Geometry check sheet. Reference: the model listing, model coordinates, mm. Round coordinates to 2 decimals unless told otherwise and drop trailing zeros. Order: outer loops, then holes, each group sorted by start corner. A loop starts at its lowest first (then second) coordinate and runs counter-clockwise, first axis right, second up. Notation, with made-up numbers: (68.5, 27) - (91.5, 27) arc R10 cw to (91.5, 37) - close; hole circle Ø2 at (-9, 11.25). An arc over 180 degrees is marked (long way). Return JSON: item names as keys, results as strings. Group by question number.
Q1. Sectioned sample at A-A, the plane z = -10.5. Record the cut outline in (x, y).
Q2. Sectioned sample at B-B, the plane x = -22.5. Record the cut outline in (y, z), then the cut area to 3 significant figures.
Q3. Gauge pin test, flat end, axial feed: pin 1 Ø2 at (x, z) = (13.644, -6.75) entering from +Y. Record the tip position at first contact, or that the pin passes through.
Q4. Sectioned sample at C-C, the plane y = 0.7. Record the cut outline in (x, z).
Q5. Sectioned sample at D-D, the plane x = -31.5. Record the cut outline in (y, z).
Q6. Material ranges on line 1 along X through (y, z) = (1.65, -6.75); line 2 along Z through (x, y) = (-22.4, 0.6); line 3 along X through (y, z) = (0.9, -3), recorded low to high.
Autodesk Inventor part; units mm, degrees
ref_plane "YZ Plane" through (0, 0, 0) normal (1, 0, 0) x (0, 1, 0)
ref_plane "XZ Plane" through (0, 0, 0) normal (0, 1, 0) x (-1, 0, 0)
ref_plane "XY Plane" through (0, 0, 0) normal (0, 0, 1) x (1, 0, 0)
sketch "Sketch1" plane through (0, 0, 0) normal (0, 1, 0) x (-1, 0, 0)
  line L0 (0, 0) -> (32.4, 0)
  line L1 (32.4, 0) -> (32.4, -13.5)
  line L2 (32.4, -13.5) -> (0, -13.5)
  line L3 (0, -13.5) -> (0, 0)
  line L4 (-5, 5) -> (37.4, 5)
  line L5 (37.4, 5) -> (37.4, -18.5)
  line L6 (37.4, -18.5) -> (-5, -18.5)
  line L7 (-5, -18.5) -> (-5, 5)
  line L8 (37.4, 5) -> (-5, 21.2758)
  line L9 (-5, 21.2758) -> (-5, -34.7758)
  line L10 (-5, -34.7758) -> (37.4, -18.5)
  line L11 (-5, 21.2758) -> (-8.0516, 15.5367)
  line L12 (-8.0516, 15.5367) -> (-17.644, 5.25)
  line L13 (-17.644, 5.25) -> (-17.644, -18.75)
  line L14 (-17.644, -18.75) -> (-8.0516, -29.0367)
  line L15 (-8.0516, -29.0367) -> (-5, -34.7758)
  point P0 (-5, -6.75)
  dimension "d0" = 32.4
  dimension "d1" = 13.5
  dimension "d2" = 5
  dimension "d5" = 21
  dimension "d6" = 21
  dimension "d8" = 28
  dimension "d9" = 28
  dimension "d11" = 6.5
  dimension "d12" = 24
  dimension "d13" = 6.5
  dimension "d15" = 165
  dimension "d16" = 165
extrude "Extrusion1" add sketch "Sketch1" along normal blind 2
fillet "Fillet1" radius 3 8 edges at (5, 1, 21.2758) (17.644, 1, 5.25) (17.644, 1, -18.75) (5, 1, -34.7758) (8.0516, 1, -29.0367) (8.0516, 1, 15.5367) (-37.4, 1, 5) (-37.4, 1, -18.5)
sketch "Sketch2" plane through (0, 2, 0) normal (0, 1, 0) x (1, 0, 0)
  circle A0 centre (3.1296, -16.2733) radius 1.1
  circle A1 centre (3.1296, 29.7733) radius 1.1
  circle A2 centre (13.644, 6.75) radius 1.1
  circle A3 centre (-22.4, -6.4734) radius 1.1
  circle A4 centre (-22.4, 19.9734) radius 1.1
  arc A5 (-35.4751, 19.2389) -> (-37.4, 16.4382) centre (-34.4, 16.4382) ccw
  line L0 (-37.4, 16.4382) -> (-37.4, -2.9382)
  arc A6 (-37.4, -2.9382) -> (-35.4751, -5.7389) centre (-34.4, -2.9382) ccw
  line L1 (-35.4751, -5.7389) -> (2.5221, -20.3247)
  arc A7 (2.5221, -20.3247) -> (6.2461, -18.9323) centre (3.5972, -17.5239) ccw
  line L2 (6.2461, -18.9323) -> (7.8661, -15.8854)
  arc A8 (8.3209, -15.2478) -> (7.8661, -15.8854) centre (10.515, -17.2938) ccw
  line L3 (8.3209, -15.2478) -> (16.8381, -6.1143)
  arc A9 (16.8381, -6.1143) -> (17.644, -4.0683) centre (14.644, -4.0683) ccw
  line L4 (17.644, -4.0683) -> (17.644, 17.5683)
  arc A10 (17.644, 17.5683) -> (16.8381, 19.6143) centre (14.644, 17.5683) ccw
  line L5 (16.8381, 19.6143) -> (8.3209, 28.7478)
  arc A11 (7.8661, 29.3854) -> (8.3209, 28.7478) centre (10.515, 30.7938) ccw
  line L6 (7.8661, 29.3854) -> (6.2461, 32.4323)
  arc A12 (6.2461, 32.4323) -> (2.5221, 33.8247) centre (3.5972, 31.0239) ccw
  line L7 (2.5221, 33.8247) -> (-35.4751, 19.2389)
  line L8 (0, 0) -> (-32.4, 0)
  line L9 (-32.4, 0) -> (-32.4, 13.5)
  line L10 (-32.4, 13.5) -> (0, 13.5)
  line L11 (0, 13.5) -> (0, 0)
  point P0 (17.644, 6.75)
  dimension "d18" = 2.2
  dimension "d19" = 2.2
  dimension "d20" = 2.2
  dimension "d21" = 2.2
  dimension "d22" = 2.2
  dimension "d23" = 4
  dimension "d25" = 15
  dimension "d26" = 4
  dimension "d27" = 4
  dimension "d28" = 4
  dimension "d29" = 4
  dimension "d30" = 4
extrude "Extrusion2" cut sketch "Sketch2" against normal up to surface (2 mm away) contours A0 | A1 | A2 | A3 | A4
equation "\"d6\" = d5"
equation "\"d9\" = d8"
equation "\"d13\" = d11"
equation "\"d16\" = d15"
equation "\"d23\" = d28"
equation "\"d26\" = d28"
equation "\"d27\" = d28"
equation "\"d29\" = d28"
equation "\"d30\" = d26"
equation "\"BendRadius\" = Thickness"
equation "\"BendReliefWidth\" = Thickness"
equation "\"BendReliefDepth\" = 0.5 * Thickness"
equation "\"CornerReliefSize\" = 4 * Thickness"
equation "\"MinimumRemnant\" = 2 * Thickness"
equation "\"TransitionRadius\" = BendRadius"
equation "\"JacobiRadiusSize\" = BendRadius"
equation "\"GapSize\" = Thickness"
properties part number "Screen Cover"
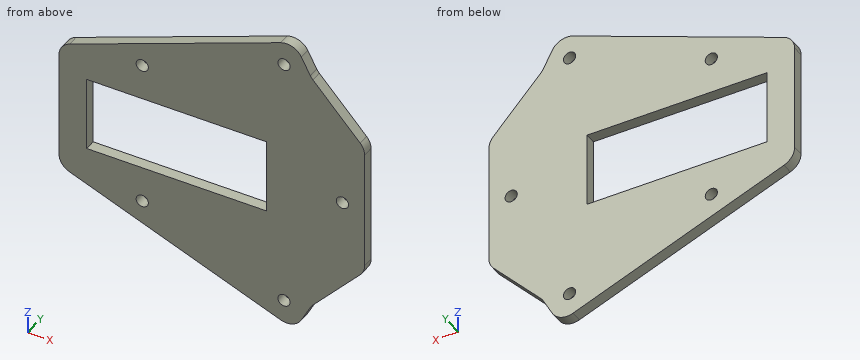
Reply:
{
 "1": {"outline": "(-37.4, 0) - (-32.4, 0) - (-32.4, 2) - (-37.4, 2) - close; (0, 0) - (17.64, 0) - (17.64, 2) - (0, 2) - close"},
 "2": {"outline": "(0, -24.22) - (2, -24.22) - (2, -21.07) - (0, -21.07) - close; (0, -18.88) - (2, -18.88) - (2, -13.5) - (0, -13.5) - close; (0, 0) - (2, 0) - (2, 5.38) - (0, 5.38) - close; (0, 7.57) - (2, 7.57) - (2, 10.72) - (0, 10.72) - close", "area": "34.1 mm^2"},
 "3": {"pin 1": "through"},
 "4": {"outline": "(-37.4, -16.44) arc R3 ccw to (-35.48, -19.24) - (2.52, -33.82) arc R3 ccw to (6.25, -32.43) - (7.87, -29.39) arc R3 cw to (8.32, -28.75) - (16.84, -19.61) arc R3 ccw to (17.64, -17.57) - (17.64, 4.07) arc R3 ccw to (16.84, 6.11) - (8.32, 15.25) arc R3 cw to (7.87, 15.89) - (6.25, 18.93) arc R3 ccw to (2.52, 20.32) - (-35.48, 5.74) arc R3 ccw to (-37.4, 2.94) - close; hole (-32.4, -13.5) - (0, -13.5) - (0, 0) - (-32.4, 0) - close; hole circle Ø2.2 at (-22.4, -19.97); hole circle Ø2.2 at (-22.4, 6.47); hole circle Ø2.2 at (3.13, -29.77); hole circle Ø2.2 at (3.13, 16.27); hole circle Ø2.2 at (13.64, -6.75)"},
 "5": {"outline": "(0, -20.76) - (2, -20.76) - (2, -13.5) - (0, -13.5) - close; (0, 0) - (2, 0) - (2, 7.26) - (0, 7.26) - close"},
 "6": {"line 1": "-37.4 to -32.4, 0 to 12.54, 14.74 to 17.64", "line 2": "-24.26 to -21.07, -18.87 to -13.5, 0 to 5.37, 7.57 to 10.76", "line 3": "-37.4 to -32.4, 0 to 17.64"}
}
